```python
from build123d import *

# Parameters (mm, degrees)
F1_DEPTH = 4
F2_R     = 3
F2_R_2   = 1.5
F3_DEPTH = 2
F4_DEPTH = 4
F5_R     = 2
F6_R     = 2
F7_R     = 2
F8_R     = 2


with BuildPart() as f1:
    # F0 (on Top) → F1 (new body)
    with BuildSketch(Plane.XY):
        Polygon((34.5, 0), (34.5, 19.5), (0, 16.5), (0, 3), align=None)
    extrude(amount=F1_DEPTH)

    # F2 (on face) → F3 (cut)
    with BuildSketch(Plane.XY.offset(4)):
        with Locations((16.5, 9.75)):
            Circle(F2_R)
        with Locations((16.5, 9.75)):
            Circle(F2_R_2, mode=Mode.SUBTRACT)
    extrude(amount=-F3_DEPTH, mode=Mode.SUBTRACT)

    # F4 (cut): a face of the model
    f4_faces = [f1.faces().sort_by_distance(p)[0] for p in [
        (16.5, 9.75, 4),
    ]]
    extrude(f4_faces, amount=-F4_DEPTH, mode=Mode.SUBTRACT)

    # F5
    f5_edges = [f1.edges().sort_by_distance(p)[0] for p in [
        (34.5, 0, 2),
    ]]
    fillet(f5_edges, radius=F5_R)

    # F6
    f6_edges = [f1.edges().sort_by_distance(p)[0] for p in [
        (34.5, 19.5, 2),
    ]]
    fillet(f6_edges, radius=F6_R)

    # F7
    f7_edges = [f1.edges().sort_by_distance(p)[0] for p in [
        (0, 16.5, 2),
    ]]
    fillet(f7_edges, radius=F7_R)

    # F8
    f8_edges = [f1.edges().sort_by_distance(p)[0] for p in [
        (0, 3, 2),
    ]]
    fillet(f8_edges, radius=F8_R)


solid = f1.part
```
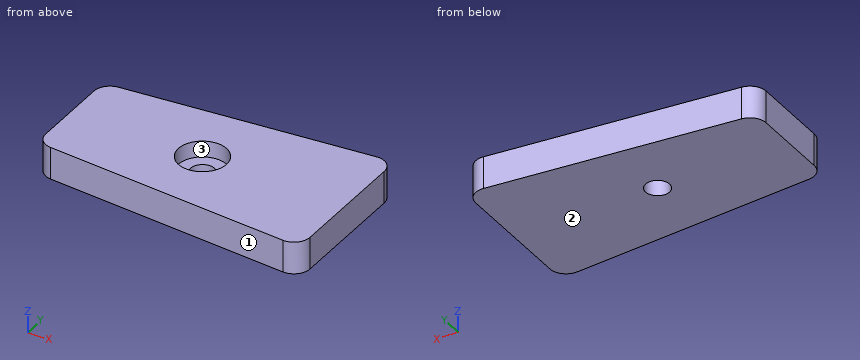
Geometry: final body of the model. Coordinates: model frame, mm. Face numbers are marked on the shaded views. Round coordinates to 2 decimals unless told otherwise and drop trailing zeros. Order: outer loops, then holes, each group sorted by start corner. A loop starts at its lowest first (then second) coordinate and runs counter-clockwise, first axis right, second up. Notation, with made-up numbers: (33.5, 36.25) - (46.5, 36.25) arc R21 cw to (46.5, 60.25) - close; hole circle Ø9 at (-19.75, 23). An arc over 180 degrees is marked (long way). Write item = value, one per line. Start each with the question number.
Q1. Cut plane D-D on y = 7.5. Return the cut outline in (x, z), and give its area (3 significant figures).
Q2. Ray query, line 1 (Y direction, x = 16.5, z = 2.65); line 2 (X direction, y = 4.75, z = 2.35); line 3 (Y direction, x = 30, z = 0.8). Return the intervals inside material, ascending. Write a range as from..to.
Q3. Pin query (flat end, axial travel): pin 1 (2 mm diameter, centred on x = 16, y = 9, fed in from +Z); pin 2 (1.5 mm diameter, centred on x = 12.5, z = 0.5, fed in from +Y). Return the tip coordinate at first contact, or that it passes through.
Q4. Cut plane A-A on z = 2.7. Return the cut outline in (x, y).
Q5. Cut plane C-C on y = 9.75. Return the cut outline in (x, z).
Q6. Cut plane B-B on x = 16.5. Return the cut outline in (y, z).
Q7. Pull-direction query (Y, two-part tool) for the marked faces 1, 2 and 3; classes: +Y half, -Y half, draft (parallel to the pull), parting line (faces both ways), or undercut.
Outcome:
q1.outline = (0, 0) - (34.5, 0) - (34.5, 4) - (18.48, 4) - (18.48, 2) - (14.52, 2) - (14.52, 4) - (0, 4) - close
q1.area = 130 mm^2
q2.line_1 = 1.57..6.75, 12.75..17.93
q2.line_2 = 0..34.5
q2.line_3 = 0.39..19.11
q3.pin_1 = 2
q3.pin_2 = 17.65
q4.outline = (0, 4.83) arc R2 ccw to (1.83, 2.84) - (32.33, 0.19) arc R2 ccw to (34.5, 2.18) - (34.5, 17.32) arc R2 ccw to (32.33, 19.31) - (1.83, 16.66) arc R2 ccw to (0, 14.67) - close; hole circle Ø6 at (16.5, 9.75)
q5.outline = (0, 0) - (15, 0) - (15, 2) - (13.5, 2) - (13.5, 4) - (0, 4) - close; (18, 0) - (34.5, 0) - (34.5, 4) - (19.5, 4) - (19.5, 2) - (18, 2) - close
q6.outline = (1.57, 0) - (8.25, 0) - (8.25, 2) - (6.75, 2) - (6.75, 4) - (1.57, 4) - close; (11.25, 0) - (17.93, 0) - (17.93, 4) - (12.75, 4) - (12.75, 2) - (11.25, 2) - close
q7.face_1 = -Y half
q7.face_2 = draft
q7.face_3 = undercut
